Solid Edge part; units mm, degrees
sketch "Sketch1" plane through (0, 0, 0) normal (0, 0, 1) x (1, 0, 0)
  circle A0 centre (0, 0) radius 10
  circle A1 centre (-12.9904, -7.5) radius 1.5
  circle A2 centre (12.9904, -7.5) radius 1.5
  circle A3 centre (-84, -80) radius 2
  circle A4 centre (-84, 80) radius 2
  circle A5 centre (84, 80) radius 2
  circle A6 centre (84, -80) radius 2
  circle A7 centre (0, 15) radius 1.5
  arc A8 (-94, 84) -> (-88, 90) centre (-88, 84) cw
  line L0 (-88, 90) -> (88, 90)
  arc A9 (88, 90) -> (94, 84) centre (88, 84) cw
  line L1 (94, 84) -> (94, -84)
  arc A10 (94, -84) -> (88, -90) centre (88, -84) cw
  line L2 (88, -90) -> (-88, -90)
  arc A11 (-88, -90) -> (-94, -84) centre (-88, -84) cw
  line L3 (-94, -84) -> (-94, 84)
  dimension "D1" = 94
  dimension "D2" = 84
  dimension "D3" = 84
extrude "Protrusion1" add sketch "Sketch1" along normal blind 5
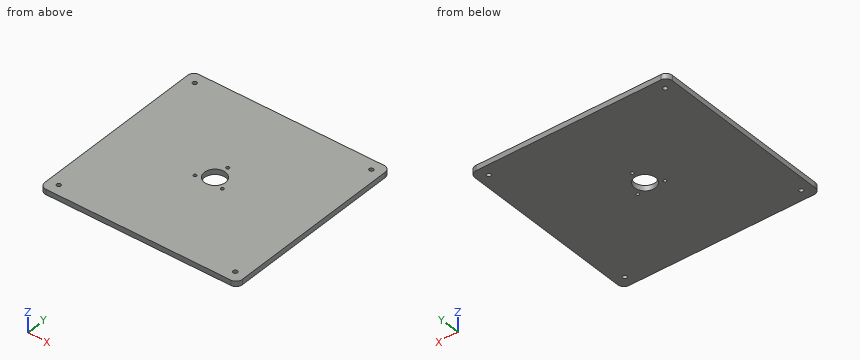
Geometry check sheet. Reference: the model listing, model coordinates, mm. Give positions to 0.01 mm unless a question says otherwise; leave off trailing zeros. Write each loop counter-clockwise with the first axis right and the second up, starting at its lowest first coordinate (ties: lowest second). Pieces come first, ordered by that corner, then holes. Notation, with made-up numbers: M 36,14 L 41,14 A25 cw 41,31 Z; hole C -26,-8.75 d4. An arc over 180 degrees is marked long. One line per question, with ' | ' between items.
1. Scan lines: line 1 along Y through (x, z) = (84, 3.75); line 2 along Y through (x, z) = (-7.5, 2.45); line 3 along Y through (x, z) = (7, 4.05). Record each from-to range of solid material in increasing order. Write a range as from..to.
Ans:
line 1: -90..-82, -78..78, 82..90 | line 2: -90..-6.61, 6.61..90 | line 3: -90..-7.14, 7.14..90
2. Cross-section at A-A (y = 0). Enter the section's corners in (x, z), plus the area to 3 significant figures.
Ans:
outline: M -94,0 L -10,0 L -10,5 L -94,5 Z; M 10,0 L 94,0 L 94,5 L 10,5 Z | area: 840 mm2
3. Gauge pin test, flat end, axial feed: pin 1 (4 mm diameter, centred on x = -66, y = 2.5, fed in from -Z). Record the tip position at first contact, or that the pin passes through.
Ans:
pin 1: z = 0
